```python
from build123d import *

# Parameters (mm, degrees)
SKETCH1_R           = 19.85
BOSS_EXTRUDE1_DEPTH = 10
SKETCH2_R           = 11.75
CUT_EXTRUDE1_DEPTH  = 10
SKETCH3_R           = 1.6
CUT_EXTRUDE2_DEPTH  = 27
SKETCH4_R           = 2.1
CUT_EXTRUDE3_DEPTH  = 10
SKETCH5_R           = 3.5
CUT_EXTRUDE4_DEPTH  = 3.5


with BuildPart() as part:
    # Sketch1 → Boss-Extrude1 (new body)
    with BuildSketch(Plane.XY):
        with BuildLine():
            Line((-34, 28), (1.418583132, 25.961381575))
            ThreePointArc((1.418583132, 25.961381575), (26.000109834, 0), (1.418583132, -25.961381575))
            Line((1.418583132, -25.961381575), (-34, -28))
            Line((-34, -28), (-44, -27))
            Line((-44, -27), (-44, 27))
            Line((-44, 27), (-34, 28))
        make_face()
        Circle(SKETCH1_R, mode=Mode.SUBTRACT)
    extrude(amount=BOSS_EXTRUDE1_DEPTH)

    # Sketch2 → Cut-Extrude1 (cut)
    with BuildSketch(Plane.XY.offset(10)):
        with Locations((-42.5, 0)):
            Circle(SKETCH2_R)
    extrude(amount=-CUT_EXTRUDE1_DEPTH, mode=Mode.SUBTRACT)

    # Sketch3 → Cut-Extrude2 (cut, symmetric)
    with BuildSketch(Plane(origin=(0, 0, 0), x_dir=(1, 0, 0), z_dir=(0, 1, 0))):
        with Locations(Location((0, -5, 0), (0, 0, 270))):
            Circle(SKETCH3_R)
    extrude(amount=CUT_EXTRUDE2_DEPTH, both=True, mode=Mode.SUBTRACT)

    # Sketch4 → Cut-Extrude3 (cut)
    with BuildSketch(Plane.XY.offset(10)):
        with Locations((-39, 22)):
            Circle(SKETCH4_R)
        with Locations((-39, -22)):
            Circle(SKETCH4_R)
    extrude(amount=-CUT_EXTRUDE3_DEPTH, mode=Mode.SUBTRACT)

    # Sketch5 → Cut-Extrude4 (cut)
    with BuildSketch(Plane.XY.offset(10)):
        with Locations((-39, 22)):
            Circle(SKETCH5_R)
        with Locations((-39, -22)):
            Circle(SKETCH5_R)
    extrude(amount=-CUT_EXTRUDE4_DEPTH, mode=Mode.SUBTRACT)


solid = part.part
```
Geometry check sheet. Reference: the model listing, model coordinates, mm. A direction names the side the tool comes from. Coordinates: 2 decimals unless noted, no trailing zeros. Loops run counter-clockwise (first coordinate to the right, second up) from the corner with the lowest first, then second, coordinate; pieces in that order, holes last. Notation, with made-up numbers: (21, 51) - (53, 51) arc R18 ccw to (53, 62) - close; hole circle Ø8 at (73, 47). An arc over 180 degrees is marked (long way). One line per item, written item: value. Start each with the question number.
(1) Cross-section at B-B on z = 2.5. Enter the section's corners in (x, y), plus the area to 3 significant figures.
(2) Cross-section at C-C on x = -39. Enter the section's corners in (y, z).
(3) Depth check by flat-ended pin: P1, Ø1, axis at x = 3, z = 5.5, coming from the +Y side; P2, Ø5.5, axis at x = -39, y = 22, coming from the +Z side; P3, Ø5, axis at x = -24.5, z = 8.5, coming from the -Y side. Enter the tip coordinate at first touch or a pass-through.
(4) Cross-section at A-A on y = 0. Enter the section's corners in (x, z), plus the area to 3 significant figures.
(5) Tool access check on faces 1 (the flat face through (-37, 20, 6.5)), 2 (the flat face through (-38.93, -27.507, 4.93)). Record the directions out of +Z, -Z, +X, -X, +Y, -Y that give a thin tool (end or side, any length) a straight path to the whole face; none if there is none.
(6) Material ranges on line 1 (Y direction, x = -39, z = 3.25); line 2 (Y direction, x = -39, z = 7.95); line 3 (X direction, y = -4, z = 1.5), recorded low to high. Write a range as [from, to].
(7) Cross-section at D-D on y = -22. Enter the section's corners in (x, z).
(8) Mould release check, pull along Y, two halves, no side actions. Record for faces 3 (the cylindrical face through (25.994, 0.552, 4.93)), 4 (the cylindrical face through (-30.753, -0.279, 5.07)), 5 (the flat face through (-44, -19, 5)): released by +Y, released by -Y, zero draft, split by the parting line, or undercut.
Results below:
1. outline: (-44, -27) - (-34, -28) - (1.42, -25.96) arc R26 ccw to (1.42, 25.96) - (-34, 28) - (-44, 27) - (-44, 11.65) arc R11.75 cw (long way) to (-44, -11.65) - close; hole circle Ø4.2 at (-39, -22); hole circle Ø4.2 at (-39, 22); hole circle Ø39.7 at (0, 0)
1. area: 1,930 mm2
2. outline: (-27.5, 0) - (-24.1, 0) - (-24.1, 6.5) - (-25.5, 6.5) - (-25.5, 10) - (-27.5, 10) - close; (-19.9, 0) - (-11.22, 0) - (-11.22, 10) - (-18.5, 10) - (-18.5, 6.5) - (-19.9, 6.5) - close; (11.22, 0) - (19.9, 0) - (19.9, 6.5) - (18.5, 6.5) - (18.5, 10) - (11.22, 10) - close; (24.1, 0) - (27.5, 0) - (27.5, 10) - (25.5, 10) - (25.5, 6.5) - (24.1, 6.5) - close
3. P1: stops at y = 25.88
3. P2: stops at z = 6.5
3. P3: stops at y = -27.6
4. outline: (-30.75, 0) - (-19.85, 0) - (-19.85, 10) - (-30.75, 10) - close; (19.85, 0) - (26, 0) - (26, 10) - (19.85, 10) - close
4. area: 171 mm2
5. face 1: +Z
5. face 2: +Z, -Z, -X, -Y
6. line 1: y = [-27.5, -24.1], [-19.9, -11.22], [11.22, 19.9], [24.1, 27.5]
6. line 2: y = [-27.5, -25.5], [-18.5, -11.22], [11.22, 18.5], [25.5, 27.5]
6. line 3: x = [-31.45, -19.44], [19.44, 25.69]
7. outline: (-44, 0) - (-41.1, 0) - (-41.1, 6.5) - (-42.5, 6.5) - (-42.5, 10) - (-44, 10) - close; (-36.9, 0) - (13.86, 0) - (13.86, 10) - (-35.5, 10) - (-35.5, 6.5) - (-36.9, 6.5) - close; hole circle Ø3.2 at (0, 5)
8. face 3: split by the parting line
8. face 4: undercut
8. face 5: zero draft
